Can you work these out from the model? Positions are in its coordinate system, mm. A direction names the side the tool comes from. Give positions to 0.01 mm unless a question says otherwise; leave off trailing zeros. Order: outer loops, then holes, each group sorted by start corner. A loop starts at its lowest first (then second) coordinate and runs counter-clockwise, first axis right, second up. Notation, with made-up numbers: (-5.75, 81) - (25.25, 81) arc R11 ccw to (25.25, 101) - close; hole circle Ø3 at (23, 10). An arc over 180 degrees is marked (long way). One line per question, with ' | ' between items.
```python
from build123d import *

# Parameters (mm, degrees)
SKETCH1_W                 = 38.1
SKETCH1_H                 = 38.1
BOSS_EXTRUDE1_DEPTH       = 3.175
F_8_CLEARANCE_HOLE1_D     = 4.4958
F_8_CLEARANCE_HOLE1_DEPTH = 10.16
F_8_CLEARANCE_HOLE1_TIP   = 1.350674586
SKETCH4_W                 = 3.175
SKETCH4_H                 = 3.175
CUT_EXTRUDE1_DEPTH        = 3.175


with BuildPart() as part:
    # Sketch1 → Boss-Extrude1 (new body)
    with BuildSketch(Plane.XY):
        Rectangle(SKETCH1_W, SKETCH1_H)
    extrude(amount=BOSS_EXTRUDE1_DEPTH)

    # #8 Clearance Hole1
    with Locations(Plane.XY.offset(3.175)):
        with Locations((0, 0)):
            Hole(F_8_CLEARANCE_HOLE1_D / 2, depth=F_8_CLEARANCE_HOLE1_DEPTH)
            with Locations((0, 0, -(F_8_CLEARANCE_HOLE1_DEPTH + F_8_CLEARANCE_HOLE1_TIP / 2))):  # 118° drill point
                Cone(0, F_8_CLEARANCE_HOLE1_D / 2, F_8_CLEARANCE_HOLE1_TIP, mode=Mode.SUBTRACT)

    # Sketch4 → Cut-Extrude1 (cut)
    with BuildSketch(Plane.XY.offset(3.175)):
        with Locations((-7.9375, 0)):
            Rectangle(SKETCH4_W, SKETCH4_H)
        with Locations((7.9375, 0)):
            Rectangle(SKETCH4_W, SKETCH4_H)
    extrude(amount=-CUT_EXTRUDE1_DEPTH, mode=Mode.SUBTRACT)


solid = part.part
```
(1) Will this pin go through, and if not, where does the flat tip stop? pin 1 (2.5 mm diameter, centred on x = 0, y = 0, fed in from +Z).
Answer below:
pin 1: through
(2) Imagine slicing it at C-C (z = 0.85). Count the separate pieces of the cut face and the enclosed holes in it, and give its area (3 significant figures).
Answer below:
separate pieces: 1 | enclosed holes: 3 | area: 1,420 mm^2
(3) On a 3-axis mill with a long thin cutter (end or side, diameter ignored), from which of +Z, -Z, +X, -X, +Y, -Y can I reach the whole of each face in a straight line? I mean faces 1 (the face through (0, 19.05, 2)), 2 (the face through (9.525, 0, 2)). Say none if no direction works.
Answer below:
face 1: +Z, -Z, +X, -X, +Y | face 2: +Z, -Z
(4) If I drill on line 1 (Y direction, x = 0, z = 2.45); line 2 (Y direction, x = -6.5, z = 1.95); line 3 (X direction, y = 1.5, z = 0.25) (3 decimals), over which ranges is the centre line in solid material (lowest first)?
Answer below:
line 1: -19.05 to -2.25, 2.25 to 19.05 | line 2: -19.05 to -1.59, 1.59 to 19.05 | line 3: -19.05 to -9.525, -6.35 to -1.674, 1.674 to 6.35, 9.525 to 19.05
(5) Imagine slicing it at B-B (y = 0). List the corners of the cut face in (x, z) for me (3 decimals).
Answer below:
outline: (-19.05, 0) - (-9.525, 0) - (-9.525, 3.175) - (-19.05, 3.175) - close; (-6.35, 0) - (-2.248, 0) - (-2.248, 3.175) - (-6.35, 3.175) - close; (2.248, 0) - (6.35, 0) - (6.35, 3.175) - (2.248, 3.175) - close; (9.525, 0) - (19.05, 0) - (19.05, 3.175) - (9.525, 3.175) - close
(6) If we mould it in two halves opening along X, with no side actions, what happens to faces 3 (the face through (-9.525, 0, 2)), 4 (the face through (-19.05, 0, 2)), 5 (the face through (4, 0, 3.175))? For each: released by +X, released by -X, zero draft, split by the parting line, or undercut.
Answer below:
face 3: undercut | face 4: released by -X | face 5: zero draft
(7) Imagine slicing it at D-D (x = 0). List the corners of the cut face in (y, z) for me (3 decimals).
Answer below:
outline: (-19.05, 0) - (-2.248, 0) - (-2.248, 3.175) - (-19.05, 3.175) - close; (2.248, 0) - (19.05, 0) - (19.05, 3.175) - (2.248, 3.175) - close
